from build123d import *

# Parameters (mm, degrees)
F1_DEPTH = 25.4
F2_R     = 6.35
F3_DEPTH = 25.4
F6_DEPTH = 25.4


with BuildPart() as f1:
    # F0 (on Front) → F1 (new body)
    with BuildSketch(Plane.XZ):
        Polygon((-46.874787, 58.363431), (-59.574787, 58.363431), (-59.574787, 7.563431), (-2.424787, 7.563431), (-2.424787, 20.263431), (-46.874787, 20.263431), align=None)
    extrude(amount=F1_DEPTH)

    # F2 (on face) → F3 (cut)
    with BuildSketch(Plane.XY.offset(20.263431)):
        with Locations((-34.174787, -12.7)):
            Circle(F2_R)
        with Locations((-15.124787, -12.7)):
            Circle(F2_R)
        with BuildLine():
            ThreePointArc((-15.124787, 0), (-6.14453, -3.719744), (-2.424787, -12.7))
            Line((-2.424787, -12.7), (-2.424787, 0))
            Line((-2.424787, 0), (-15.124787, 0))
        make_face()
        with BuildLine():
            ThreePointArc((-2.424787, -12.7), (-6.14453, -21.680256), (-15.124787, -25.4))
            Line((-15.124787, -25.4), (-2.424787, -25.4))
            Line((-2.424787, -25.4), (-2.424787, -12.7))
        make_face()
    extrude(amount=-F3_DEPTH, mode=Mode.SUBTRACT)

    # F4 (on face) → F6 (cut)
    with BuildSketch(Plane.YZ.offset(-46.874787)):
        with BuildLine():
            ThreePointArc((-19.517475, 45.663431), (-13.167475, 39.313431), (-6.817475, 45.663431))
            ThreePointArc((-6.817475, 45.663431), (-13.167475, 52.013431), (-19.517475, 45.663431))
        make_face()
        with BuildLine():
            ThreePointArc((-19.517475, 45.663431), (-13.167475, 52.013431), (-6.817475, 45.663431))
            Line((-6.817475, 45.663431), (-6.817475, 58.363431))
            Line((-6.817475, 58.363431), (-19.517475, 58.363431))
            Line((-19.517475, 58.363431), (-19.517475, 45.663431))
        make_face()
    extrude(amount=-F6_DEPTH, mode=Mode.SUBTRACT)


solid = f1.part
Here's how the part is built. I have some questions about the finished solid (model axes, mm). A direction names the side the tool comes from. Round coordinates to 2 decimals unless told otherwise and drop trailing zeros. Order: outer loops, then holes, each group sorted by start corner. A loop starts at its lowest first (then second) coordinate and runs counter-clockwise, first axis right, second up. Notation, with made-up numbers: M 30,-8 L 41,-8 A11 ccw 41,1 Z; hole C 13.5,2.25 d11. An arc over 180 degrees is marked long. One line per question, with ' | ' between items.
1) Imagine slicing it at C-C, the plane y = -11.75. Write out the boundary of the cut face in (x, z), plus the area to 3 significant figures.
Checked values:
outline: M -59.57,7.56 L -40.45,7.56 L -40.45,20.26 L -46.87,20.26 L -46.87,39.47 L -59.57,39.47 Z; M -27.9,7.56 L -21.4,7.56 L -21.4,20.26 L -27.9,20.26 Z; M -8.85,7.56 L -2.46,7.56 L -2.46,20.26 L -8.85,20.26 Z | area: 650 mm²
2) Imagine slicing it at D-D, the plane x = -52. Write out the boundary of the cut face in (y, z), plus the area to 3 significant figures.
Checked values:
outline: M -25.4,7.56 L 0,7.56 L 0,58.36 L -6.82,58.36 L -6.82,45.66 A6.35 cw -19.52,45.66 L -19.52,58.36 L -25.4,58.36 Z | area: 1,070 mm²
3) Imagine slicing it at A-A, the plane z = 16.5. Write out the boundary of the cut face in (x, y), plus the area to 3 significant figures.
Checked values:
outline: M -59.57,-25.4 L -15.12,-25.4 A12.7 ccw -2.42,-12.7 A12.7 ccw -15.12,0 L -59.57,0 Z; hole C -34.17,-12.7 d12.7; hole C -15.12,-12.7 d12.7 | area: 1,130 mm²
4) On a 3-axis mill with a long thin cutter (end or side, diameter ignored), from which of +Z, -Z, +X, -X, +Y, -Y can I reach the whole of each face in a straight line? I mean faces 1 (the flat face through (-53, -6.817, 52)), 2 (the flat face through (-46.875, -13, 35)), 3 (the flat face through (-48, 0, 28)). Say none if no direction works.
Checked values:
face 1: +Z, +X, -X | face 2: +Z, +X, +Y, -Y | face 3: +Z, -Z, +X, -X, +Y
5) Imagine slicing it at B-B, the plane x = -20. Write out the boundary of the cut face in (y, z), plus the area to 3 significant figures.
Checked values:
outline: M -25.4,7.56 L -16.77,7.56 L -16.77,20.26 L -25.4,20.26 Z; M -8.63,7.56 L 0,7.56 L 0,20.26 L -8.63,20.26 Z | area: 219 mm²
6) I'm going to push flat-ended pins straight in: pin 1 Ø3 at (y, z) = (-3.5, 16.5) entering from +X; pin 2 Ø5 at (y, z) = (-3.5, 18) entering from +X; pin 3 Ø12 at (x, y) = (-12.5, -3.5) entering from +Z; pin 4 Ø11.5 at (x, y) = (-15.12, -12.7) entering from -Z. Where does each tip first touch, or does it pass through?
Checked values:
pin 1: stops at x = -5.03 | pin 2: stops at x = -4.34 | pin 3: stops at z = 20.26 | pin 4: passes through
7) We'd pull the mould along Y, two halves only. Please class faces 4 (the cylindrical face through (-31.24, -18.33, 14)), 5 (the flat face through (-48, -25.4, 28)), 6 (the flat face through (-31, -7, 7.563)): released by +Y, released by -Y, zero draft, split by the parting line, or undercut.
Checked values:
face 4: undercut | face 5: released by -Y | face 6: zero draft
8) I need wall thicknesses on line 1 (Y direction, x = -47.5, z = 46.5); line 2 (Z direction, x = -11.5, y = -3); line 3 (X direction, y = -13, z = 38). Which ranges of each line are inside material? Lowest first, please.
Checked values:
line 1: y = -25.4 to -19.52, -6.82 to 0 | line 2: z = 7.56 to 20.26 | line 3: x = -59.57 to -46.87
